```python
from build123d import *

# Parameters (mm, degrees)
BOSS_EXTRUDE1_DEPTH = 76.2
CUT_EXTRUDE1_DEPTH  = 10
SKETCH4_R           = 10
SKETCH4_R_2         = 12.7
CUT_EXTRUDE2_DEPTH  = 10


with BuildPart() as part:
    # Sketch2 → Boss-Extrude1 (new body, symmetric)
    with BuildSketch(Plane.XY):
        with BuildLine():
            Line((-38.1, 0), (38.1, 0))
            Line((38.1, 0), (38.1, 76.2))
            Line((38.1, 76.2), (34.925, 76.2))
            ThreePointArc((34.925, 76.2), (32.67993597, 75.27006403), (31.75, 73.025))
            Line((31.75, 73.025), (31.75, 9.525))
            ThreePointArc((31.75, 9.525), (30.82006403, 7.27993597), (28.575, 6.35))
            Line((28.575, 6.35), (-34.925, 6.35))
            ThreePointArc((-34.925, 6.35), (-37.17006403, 5.42006403), (-38.1, 3.175))
            Line((-38.1, 3.175), (-38.1, 0))
        make_face()
    extrude(amount=BOSS_EXTRUDE1_DEPTH, both=True)

    # Sketch3 → Cut-Extrude1 (cut)
    with BuildSketch(Plane(origin=(38.1, 0, 0), x_dir=(0, 0, -1), z_dir=(1, 0, 0))):
        with BuildLine():
            Line((-28.25, 65.4), (-28.25, 14.6))
            ThreePointArc((-28.25, 14.6), (-31.75, 11.1), (-35.25, 14.6))
            Line((-35.25, 14.6), (-35.25, 65.4))
            ThreePointArc((-35.25, 65.4), (-31.75, 68.9), (-28.25, 65.4))
        make_face()
        with BuildLine():
            Line((28.25, 65.4), (28.25, 14.6))
            ThreePointArc((28.25, 14.6), (31.75, 11.1), (35.25, 14.6))
            Line((35.25, 14.6), (35.25, 65.4))
            ThreePointArc((35.25, 65.4), (31.75, 68.9), (28.25, 65.4))
        make_face()
        with BuildLine():
            Line((3.5, 65.4), (3.5, 14.6))
            ThreePointArc((3.5, 14.6), (0, 11.1), (-3.5, 14.6))
            Line((-3.5, 14.6), (-3.5, 65.4))
            ThreePointArc((-3.5, 65.4), (0, 68.9), (3.5, 65.4))
        make_face()
    extrude(amount=-CUT_EXTRUDE1_DEPTH, mode=Mode.SUBTRACT)

    # Sketch4 → Cut-Extrude2 (cut)
    with BuildSketch(Plane.XZ):
        Circle(SKETCH4_R)
        with Locations((0, 52.5)):
            Circle(SKETCH4_R_2)
        with Locations((0, -52.5)):
            Circle(SKETCH4_R_2)
    extrude(amount=-CUT_EXTRUDE2_DEPTH, mode=Mode.SUBTRACT)


solid = part.part
```
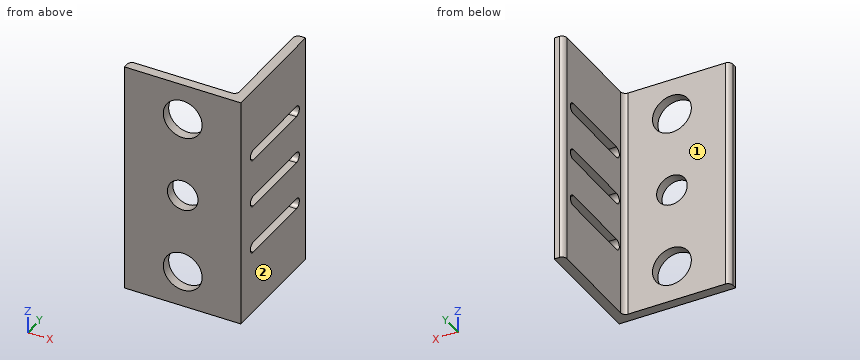
Build history of the part. All positions in model axes, mm. Face numbers are marked on the shaded views. A direction names the side the tool comes from. Coordinates: 2 decimals unless noted, no trailing zeros. Order: outer loops, then holes, each group sorted by start corner. A loop starts at its lowest first (then second) coordinate and runs counter-clockwise, first axis right, second up. Notation, with made-up numbers: M 79,54.5 L 133,54.5 A27 ccw 133,91.5 Z; hole C 77.25,42 d2. An arc over 180 degrees is marked long. One line per question, with ' | ' between items. Start each with the question number.
1. Cut at D-D (z = 31.75). Write the cut outline in (x, y) (3 decimals).
2. Wall check: line 1 along Z through (x, y) = (0, 1.5); line 2 along X through (y, z) = (10, 39); line 3 along Y through (x, z) = (22, -9). Give the ranges that are in metal, low to high. Write a range as [from, to].
3. Cut at B-B (z = 0). Write the cut outline in (x, y) (3 decimals).
4. Flat gauge pins, fed straight in: P1, Ø2, axis at y = 27, z = -15.5, coming from the -X side; P2, Ø18, axis at x = 0, z = 0, coming from the +Y side; P3, Ø8, axis at x = 5.5, z = 60, coming from the +Y side. Where does each tip first touch, or does it go through?
5. Cut at C-C (x = 0). Write the cut outline in (y, z).
6. Cut at A-A (y = 32.5). Write the cut outline in (x, z).
7. Tool access for the marked faces 1 and 2: list every direction of +Z, -Z, +X, -X, +Y, -Y with a clear straight run to the whole face (end or side of a thin tool).
The answers:
1) outline: M -38.1,0 L 38.1,0 L 38.1,11.1 L 31.75,11.1 L 31.75,9.525 A3.175 cw 28.575,6.35 L -34.925,6.35 A3.175 ccw -38.1,3.175 Z; M 31.75,68.9 L 38.1,68.9 L 38.1,76.2 L 34.925,76.2 A3.175 ccw 31.75,73.025 Z
2) line 1: z = [-76.2, -65.2], [-39.8, -10], [10, 39.8], [65.2, 76.2] | line 2: x = [31.75, 38.1] | line 3: y = [0, 6.35]
3) outline: M -38.1,0 L -10,0 L -10,6.35 L -34.925,6.35 A3.175 ccw -38.1,3.175 Z; M 10,0 L 38.1,0 L 38.1,11.1 L 31.75,11.1 L 31.75,9.525 A3.175 cw 28.575,6.35 L 10,6.35 Z; M 31.75,68.9 L 38.1,68.9 L 38.1,76.2 L 34.925,76.2 A3.175 ccw 31.75,73.025 Z
4) P1: stops at x = 31.75 | P2: passes through | P3: stops at y = 6.35
5) outline: M 0,-76.2 L 6.35,-76.2 L 6.35,-65.2 L 0,-65.2 Z; M 0,-39.8 L 6.35,-39.8 L 6.35,-10 L 0,-10 Z; M 0,10 L 6.35,10 L 6.35,39.8 L 0,39.8 Z; M 0,65.2 L 6.35,65.2 L 6.35,76.2 L 0,76.2 Z
6) outline: M 31.75,-76.2 L 38.1,-76.2 L 38.1,-35.25 L 31.75,-35.25 Z; M 31.75,-28.25 L 38.1,-28.25 L 38.1,-3.5 L 31.75,-3.5 Z; M 31.75,3.5 L 38.1,3.5 L 38.1,28.25 L 31.75,28.25 Z; M 31.75,35.25 L 38.1,35.25 L 38.1,76.2 L 31.75,76.2 Z
7) face 1: +Z, -Z, -X, +Y | face 2: +Z, -Z, +X, +Y, -Y
